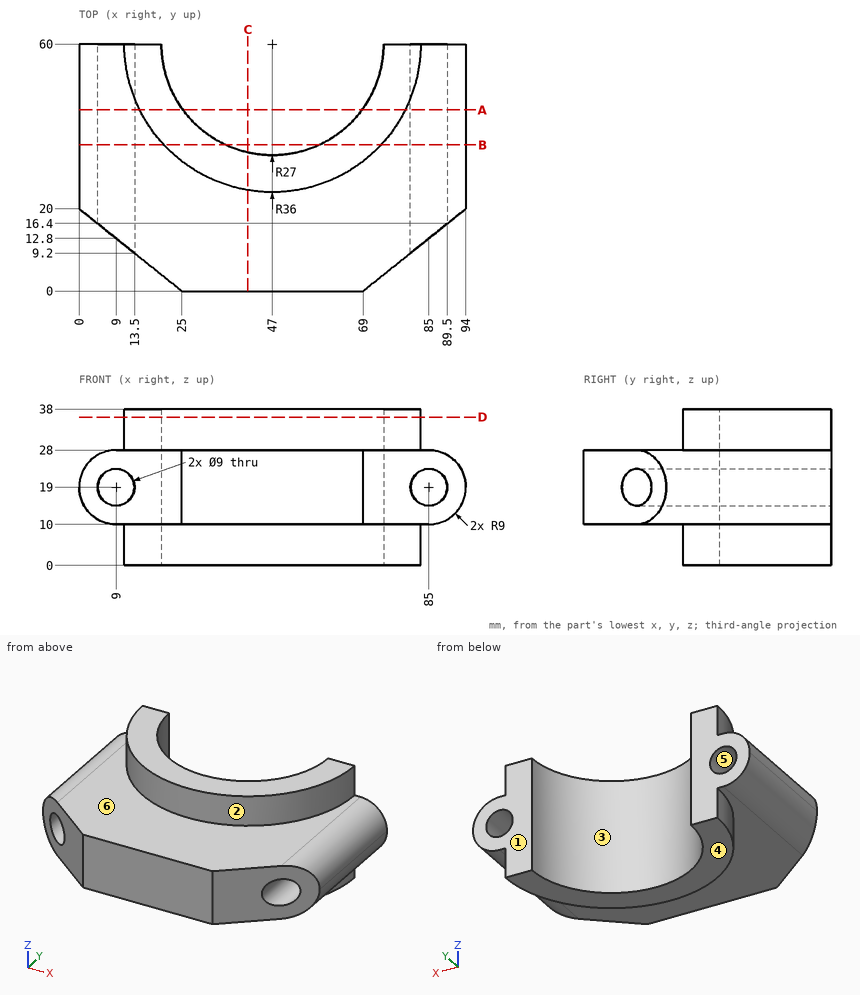
Geometry check sheet. Reference: drawing and pictorial views, mm from the part's lowest x, y, z. A direction names the side the tool comes from. Give positions to 0.01 mm unless a question says otherwise; leave off trailing zeros. Loops run counter-clockwise (first coordinate to the right, second up) from the corner with the lowest first, then second, coordinate; pieces in that order, holes last.
1. Section check D-D, the plane z = 36. Enter the section's corners in (x, y).
2. Section check B-B, the plane y = 35.5. Enter the section's corners in (x, z), then the cut area to 3 significant figures.
3. Section check A-A, the plane y = 44. Enter the section's corners in (x, z), then the cut area to 3 significant figures.
4. Go/stop test with flat-tipped pins: pin 1 Ø3 at (x, z) = (20.5, 5.5) entering from -Y; pin 2 Ø5 at (y, z) = (16, 28.5) entering from +X; pin 3 Ø4 at (y, z) = (37.5, 9) entering from -X. Record where each tip stops, or that it passes through.
5. Mould release check, pull along Z, two halves, no side actions. Record for the marked faces 3, 4, 5 and 6: released by +Z, released by -Z, zero draft, split by the parting line, or undercut.
6. Set-up check for the marked faces 1 and 2: record each of +Z, -Z, +X, -X, +Y, -Y from which the full face is reachable in a straight line by a thin tool's end or side.
7. Thickness scan on line 1 (Z direction, x = 9, y = 45); line 2 (X direction, y = 24.5, z = 19); line 3 (X direction, y = 43.5, z = 19). Record the ranges inside material, lowest first.
8. Section check C-C, the plane x = 41. Enter the section's corners in (y, z), then the cut area to 3 significant figures.
Geometry says:
1. outline: (11, 60) arc R36 ccw to (83, 60) - (74, 60) arc R27 cw to (20, 60) - close
2. outline: (9, 10) - (20.62, 10) - (20.62, 0) - (35.65, 0) - (35.65, 38) - (20.62, 38) - (20.62, 28) - (9, 28) arc R9 ccw to start; (58.35, 0) - (73.38, 0) - (73.38, 10) - (85, 10) arc R9 ccw to (85, 28) - (73.38, 28) - (73.38, 38) - (58.35, 38) - close; hole circle Ø9 at (9, 19); hole circle Ø9 at (85, 19)
2. area: 1,690 mm2
3. outline: (9, 10) - (14.75, 10) - (14.75, 0) - (25.25, 0) - (25.25, 38) - (14.75, 38) - (14.75, 28) - (9, 28) arc R9 ccw to start; (68.75, 0) - (79.25, 0) - (79.25, 10) - (85, 10) arc R9 ccw to (85, 28) - (79.25, 28) - (79.25, 38) - (68.75, 38) - close; hole circle Ø9 at (9, 19); hole circle Ø9 at (85, 19)
3. area: 1,130 mm2
4. pin 1: stops at y = 34.1
4. pin 2: stops at x = 90.34
4. pin 3: stops at x = 4.88
5. face 3: zero draft
5. face 4: released by -Z
5. face 5: undercut
5. face 6: released by +Z
6. face 1: +Z, -Z, +X, -X, +Y
6. face 2: +Z, -Y
7. line 1: z = 10 to 14.5, 23.5 to 28
7. line 2: x = 0 to 4.5, 13.5 to 80.5, 89.5 to 94
7. line 3: x = 0 to 4.5, 13.5 to 25.63, 68.37 to 80.5, 89.5 to 94
8. outline: (0, 10) - (24.5, 10) - (24.5, 0) - (33.68, 0) - (33.68, 38) - (24.5, 38) - (24.5, 28) - (0, 28) - close
8. area: 790 mm2
